from build123d import *

# Parameters (mm, degrees)
F0_W      = 45
F0_H      = 100
F0_R      = 2.7
F1_DEPTH  = 20
F2_W      = 1.5
F2_H      = 30
F3_DEPTH  = 25
F4_R      = 2.2
F5_DEPTH  = 25
F6_DEPTH  = 20
F7_R      = 5.2
F8_DEPTH  = 40
F9_W      = 2
F9_H      = 9
F10_DEPTH = 40
F11_W     = 2
F11_H     = 15
F12_DEPTH = 10
F13_R     = 2.2
F14_DEPTH = 25
F15_SIZE  = 10
F16_W     = 5
F16_H     = 9
F17_DEPTH = 10


# Not quite as in the source:
# - a pattern or mirror of a feature is missing from the dataset's text; its kind, count and spacing are read off the source's solid


with BuildPart() as f1:
    # F0 (on Top) → F1 (new body)
    with BuildSketch(Plane.XY):
        Rectangle(F0_W, F0_H)
        with Locations((-15, -40)):
            Circle(F0_R, mode=Mode.SUBTRACT)
        with Locations((15, -40)):
            Circle(F0_R, mode=Mode.SUBTRACT)
        with Locations((-15, 40)):
            Circle(F0_R, mode=Mode.SUBTRACT)
        with Locations((15, 40)):
            Circle(F0_R, mode=Mode.SUBTRACT)
    extrude(amount=F1_DEPTH)

    # F2 (on face) → F3 (cut)
    with BuildSketch(Plane.XY.offset(20)):
        with Locations((6.75, -35)):
            Rectangle(F2_W, F2_H)
    f3 = extrude(amount=-F3_DEPTH, mode=Mode.SUBTRACT)

    # F3_copies: F3 across plane
    add(f3.mirror(Plane.ZX), mode=Mode.SUBTRACT)

    # F4 (on face) → F5 (cut)
    with BuildSketch(Plane.YZ.offset(22.5)):
        with Locations((-46, 10)):
            Circle(F4_R)
    f5 = extrude(amount=-F5_DEPTH, mode=Mode.SUBTRACT)

    # F5_copies: F5 across plane
    add(f5.mirror(Plane.ZX), mode=Mode.SUBTRACT)

    # F6 (add): a face of the model
    f6_faces = [f1.faces().sort_by_distance(p)[0] for p in [
        (-22.5, 0, 10),
    ]]
    extrude(f6_faces, amount=F6_DEPTH)

    # F7 (on face) → F8 (cut)
    with BuildSketch(Plane(origin=(-42.5, 0, 0), x_dir=(0, -1, 0), z_dir=(-1, 0, 0))):
        with Locations((-30, 10)):
            Circle(F7_R)
        with Locations((30, 10)):
            Circle(F7_R)
    extrude(amount=-F8_DEPTH, mode=Mode.SUBTRACT)

    # F9 (on face) → F10 (cut)
    with BuildSketch(Plane(origin=(-42.5, 0, 0), x_dir=(0, -1, 0), z_dir=(-1, 0, 0))):
        with Locations((-16, 4.5)):
            Rectangle(F9_W, F9_H)
        Polygon((-17, 9), (-15, 9), (-15, 11), (-30, 11), (-30, 9), align=None)
    f10 = extrude(amount=-F10_DEPTH, mode=Mode.SUBTRACT)

    # F10_copies: F10 across plane
    add(f10.mirror(Plane(origin=(0, 0, 0), x_dir=(0, 0, -1), z_dir=(0, -1, 0))), mode=Mode.SUBTRACT)

    # F11 (on face) → F12 (cut)
    with BuildSketch(Plane(origin=(0, 0, 0), x_dir=(1, 0, 0), z_dir=(0, 0, -1))):
        with Locations((-3.5, -22.5)):
            Rectangle(F11_W, F11_H)
    f12 = extrude(amount=-F12_DEPTH, mode=Mode.SUBTRACT)

    # F12_copies: F12 across plane
    add(f12.mirror(Plane(origin=(0, 0, 0), x_dir=(0, 0, -1), z_dir=(0, -1, 0))), mode=Mode.SUBTRACT)

    # F13 (on face) → F14 (cut, symmetric)
    with BuildSketch(Plane.XY.offset(9)):
        with Locations((-35.5, 20.9485298356)):
            Circle(F13_R)
        with Locations((-11.5, 20.9485298356)):
            Circle(F13_R)
        with Locations((-23.5, 20.9485298356)):
            Circle(F13_R)
    f14 = extrude(amount=F14_DEPTH, both=True, mode=Mode.SUBTRACT)

    # F14_copies: F14 across plane
    add(f14.mirror(Plane(origin=(0, 0, 0), x_dir=(0, 0, -1), z_dir=(0, -1, 0))), mode=Mode.SUBTRACT)

    # F15
    f15_edges = [f1.edges().sort_by_distance(p)[0] for p in [
        (-42.5, 50, 10),
        (-42.5, -50, 10),
    ]]
    chamfer(f15_edges, length=F15_SIZE)

    # F16 (on face) → F17 (cut)
    with BuildSketch(Plane.XZ.offset(50)):
        with Locations((-4, 10)):
            Rectangle(F16_W, F16_H)
    f17 = extrude(amount=-F17_DEPTH, mode=Mode.SUBTRACT)

    # F17_copies: F17 across plane
    add(f17.mirror(Plane.ZX), mode=Mode.SUBTRACT)


solid = f1.part
For this review, take the finished solid that the model builds, in its own axes (mm). A direction names the side the tool comes from. Round coordinates to 2 decimals unless told otherwise and drop trailing zeros. Order: outer loops, then holes, each group sorted by start corner. A loop starts at its lowest first (then second) coordinate and runs counter-clockwise, first axis right, second up. Notation, with made-up numbers: M 62,10 L 101,10 A15 ccw 101,36 Z; hole C 86.5,32.25 d3. An arc over 180 degrees is marked long. Use a Markdown table: item, result. Add a question column.
Item 1: Mouldability with a two-part tool opening along X and no side actions: class faces 4 (the cylindrical face through (15.105, 48.198, 10.097)), 5 (the cylindrical face through (-23.98, 18.8, 15.56)) as released by +X, released by -X, zero draft, split by the parting line, or undercut.
Item 2: To check wall thickness, follow line 1 along Y through (x, z) = (-15, 15.5); line 2 along Y through (x, z) = (-10, 10.5); line 3 along X through (y, z) = (-31.5, 6.75). State the ranges of each line that lie inside material, in increasing order.
Item 3: Add section A-A, the plane y = -46. Give the boundary of the cut face in (x, z).
Item 4: Insertion check: pin 1 (1.5 mm diameter, centred on x = -3, z = 12, fed in from +Y); pin 2 (3.5 mm diameter, centred on y = 46, z = 10, fed in from -X). Each pin has a flat end and moves straight along its axis. Give the tip position at first contact, or say it passes through.
Item 5: Add section B-B, the plane x = -35.5. State how many separate pieces and enclosed holes the cut face has, then the cut area to 3 significant figures.
Item 6: Tool access review of faces 1 (the flat face through (-4.5, 24, 4)), 2 (the flat face through (-24, -18, 9)), 3 (the flat face through (-4, 45, 14.5)): name each direction out of +Z, -Z, +X, -X, +Y, -Y from which nothing blocks a thin tool from reaching the whole face with its end or side.
Item 7: Add section D-D, the plane x = -15. Give the boundary of the cut face in (y, z), then the cut area to 3 significant figures.
Geometry results:
| question | item | result |
|---|---|---|
| 1 | face 4 | zero draft |
| 1 | face 5 | undercut |
| 2 | line 1 | y = -50 to -42.7, -37.3 to 37.3, 42.7 to 50 |
| 2 | line 2 | y = -50 to -35.18, -15 to 15, 35.18 to 50 |
| 2 | line 3 | x = -2.5 to 6, 7.5 to 22.5 |
| 3 | outline | M -36.5,0 L 6,0 L 6,7.8 L -1.5,7.8 L -1.5,5.5 L -6.5,5.5 L -6.5,14.5 L -1.5,14.5 L -1.5,12.2 L 6,12.2 L 6,20 L -36.5,20 Z; M 7.5,0 L 22.5,0 L 22.5,7.8 L 7.5,7.8 Z; M 7.5,12.2 L 22.5,12.2 L 22.5,20 L 7.5,20 Z |
| 4 | pin 1 | stops at y = 40 |
| 4 | pin 2 | stops at x = -38.25 |
| 5 | separate pieces | 5 |
| 5 | enclosed holes | 0 |
| 5 | area | 1,480 mm² |
| 6 | face 1 | -Z |
| 6 | face 2 | -X |
| 6 | face 3 | +Y |
| 7 | outline | M -50,0 L -42.7,0 L -42.7,20 L -50,20 Z; M -37.3,0 L -17,0 L -17,9 L -24.9,9 A5.2 cw long -24.9,11 L -15,11 L -15,0 L 15,0 L 15,11 L 24.9,11 A5.2 cw long 24.9,9 L 17,9 L 17,0 L 37.3,0 L 37.3,20 L -37.3,20 Z; M 42.7,0 L 50,0 L 50,20 L 42.7,20 Z |
| 7 | area | 1,540 mm² |
